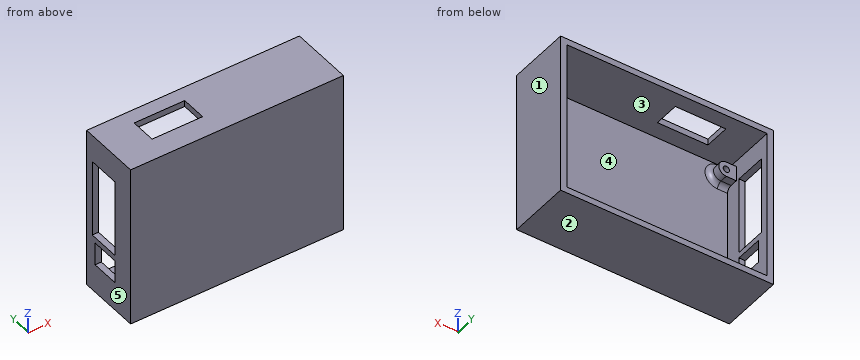
```python
from build123d import *

# Parameters (mm, degrees)
SKETCH_1_W          = 85
SKETCH_1_H          = 65
EXTRUDE_1_DEPTH     = 25
SHELL_1_T           = -2.5
SKETCH_2_R          = 3
SKETCH_2_R_2        = 1.25
EXTRUDE_2_DEPTH     = 5
SKETCH_3_W          = 20.2
SKETCH_3_H          = 10.2
CUT_EXTRUDE_1_DEPTH = 3.5
SKETCH_4_W          = 9.2
SKETCH_4_H          = 11.2
SKETCH_4_W_2        = 31
SKETCH_4_H_2        = 12.8
CUT_EXTRUDE_2_DEPTH = 3.5
FILLET_1_R          = 2


with BuildPart() as part:
    # 草图1 → 凸台-拉伸1 (new body)
    with BuildSketch(Plane(origin=(0, 0, 0), x_dir=(1, 0, 0), z_dir=(0, 1, 0))):
        Rectangle(SKETCH_1_W, SKETCH_1_H)
    extrude(amount=EXTRUDE_1_DEPTH)

    # 抽壳1
    shell_1_openings = [part.faces().sort_by_distance(p)[0] for p in [
        (0, 25, 0),
    ]]
    offset(amount=SHELL_1_T, openings=shell_1_openings, kind=Kind.INTERSECTION)

    # 草图2 → 凸台-拉伸2 (add)
    with BuildSketch(Plane(origin=(0, 2.5, 0), x_dir=(1, 0, 0), z_dir=(0, 1, 0))):
        with Locations((32.25, 24.75)):
            Circle(SKETCH_2_R)
        with Locations((32.25, 24.75)):
            Circle(SKETCH_2_R_2, mode=Mode.SUBTRACT)
        with Locations((32.25, -24.75)):
            Circle(SKETCH_2_R)
        with Locations((32.25, -24.75)):
            Circle(SKETCH_2_R_2, mode=Mode.SUBTRACT)
        with BuildLine():
            Line((-36, 27.75), (-40, 27.75))
            Line((-40, 27.75), (-40, 21.75))
            Line((-40, 21.75), (-36, 21.75))
            ThreePointArc((-36, 21.75), (-33, 24.75), (-36, 27.75))
        make_face()
        with Locations((-36, 24.75)):
            Circle(SKETCH_2_R_2, mode=Mode.SUBTRACT)
        with BuildLine():
            Line((-36, -21.75), (-40, -21.75))
            Line((-40, -21.75), (-40, -27.75))
            Line((-40, -27.75), (-36, -27.75))
            ThreePointArc((-36, -27.75), (-33, -24.75), (-36, -21.75))
        make_face()
        with Locations((-36, -24.75)):
            Circle(SKETCH_2_R_2, mode=Mode.SUBTRACT)
    extrude(amount=EXTRUDE_2_DEPTH)

    # 草图3 → 切除-拉伸1 (cut, through all)
    with BuildSketch(Plane(origin=(0, 0, 30), x_dir=(-1, 0, 0), z_dir=(0, 0, -1))):
        with Locations((17.5, 14.1)):
            Rectangle(SKETCH_3_W, SKETCH_3_H)
    extrude(amount=-CUT_EXTRUDE_1_DEPTH, mode=Mode.SUBTRACT)

    # 草图4 → 切除-拉伸2 (cut, through all)
    with BuildSketch(Plane(origin=(-40, 0, 0), x_dir=(0, 0, -1), z_dir=(1, 0, 0))):
        with Locations((16.4, 14.6)):
            Rectangle(SKETCH_4_W, SKETCH_4_H)
        with Locations((-6, 15.4)):
            Rectangle(SKETCH_4_W_2, SKETCH_4_H_2)
    extrude(amount=-CUT_EXTRUDE_2_DEPTH, mode=Mode.SUBTRACT)

    # 圆角1
    fillet_1_edges = [part.edges().sort_by_distance(p)[0] for p in [
        (29.25, 2.5, -24.75),
        (29.25, 2.5, 24.75),
        (-33, 2.5, -24.75),
        (-38, 2.5, -27.75),
        (-38, 2.5, -21.75),
        (-33, 2.5, 24.75),
        (-38, 2.5, 21.75),
        (-38, 2.5, 27.75),
    ]]
    fillet(fillet_1_edges, radius=FILLET_1_R)


solid = part.part
```
Check sheet for the modelled part. Datum: model origin and axes. Units: mm. Face numbers are marked on the shaded views. A direction names the side the tool comes from. Round coordinates to 2 decimals unless told otherwise and drop trailing zeros. Write each loop counter-clockwise with the first axis right and the second up, starting at its lowest first coordinate (ties: lowest second). Pieces come first, ordered by that corner, then holes. Notation, with made-up numbers: (86.25, 74.25) -> (123.25, 74.25) arc R23 ccw to (123.25, 99.25) -> close; hole circle Ø10 at (-31.75, -9.5). An arc over 180 degrees is marked (long way). Put each result on its own line as item: value.
(1) Sectioned sample at C-C (x = 8). Enter the section's corners in (y, z).
Values found:
outline: (0, -32.5) -> (25, -32.5) -> (25, -30) -> (2.5, -30) -> (2.5, 30) -> (25, 30) -> (25, 32.5) -> (0, 32.5) -> close
(2) Tool access check on the marked faces 4 and 5. Record the directions out of +Z, -Z, +X, -X, +Y, -Y that give a thin tool (end or side, any length) a straight path to the whole face; none if there is none.
Values found:
face 4: +Y
face 5: +Z, -Z, -X, +Y, -Y
(3) Sectioned sample at A-A (y = 15). Enter the section's corners in (x, z), plus the area to 3 significant figures.
Values found:
outline: (-42.5, -32.5) -> (42.5, -32.5) -> (42.5, 32.5) -> (-7.4, 32.5) -> (-7.4, 30) -> (40, 30) -> (40, -30) -> (-40, -30) -> (-40, -21) -> (-42.5, -21) -> close; (-42.5, -11.8) -> (-40, -11.8) -> (-40, -9.5) -> (-42.5, -9.5) -> close; (-42.5, 21.5) -> (-40, 21.5) -> (-40, 30) -> (-27.6, 30) -> (-27.6, 32.5) -> (-42.5, 32.5) -> close
area: 574 mm^2
(4) Go/stop test with flat-tipped pins: pin 1 Ø3 at (x, z) = (33.5, 24.5) entering from +Y; pin 2 Ø1.5 at (y, z) = (13, 13.5) entering from -X. Record where each tip stops, or that it passes through.
Values found:
pin 1: stops at y = 7.5
pin 2: stops at x = 40
(5) Mould release check, pull along X, two halves, no side actions. Record for the marked faces 1, 2 and 3: released by +X, released by -X, zero draft, split by the parting line, or undercut.
Values found:
face 1: released by +X
face 2: zero draft
face 3: undercut
(6) Material ranges on line 1 (Z direction, x = 32.25, y = 6.1); line 2 (X direction, y = 5.55, z = 24.75), recorded low to high.
Values found:
line 1: z = -32.5 to -30, -27.75 to -26, -23.5 to -21.75, 21.75 to 23.5, 26 to 27.75, 30 to 32.5
line 2: x = -42.5 to -37.25, -34.75 to -33, 29.25 to 31, 33.5 to 35.25, 40 to 42.5
(7) Sectioned sample at B-B (z = 9). Enter the section's corners in (x, y).
Values found:
outline: (-42.5, 0) -> (42.5, 0) -> (42.5, 25) -> (40, 25) -> (40, 2.5) -> (-40, 2.5) -> (-40, 9) -> (-42.5, 9) -> close; (-42.5, 21.8) -> (-40, 21.8) -> (-40, 25) -> (-42.5, 25) -> close
(8) Sectioned sample at D-D (z = -10.5). Enter the section's corners in (x, y), plus the area to 3 significant figures.
Values found:
outline: (-42.5, 0) -> (42.5, 0) -> (42.5, 25) -> (40, 25) -> (40, 2.5) -> (-40, 2.5) -> (-40, 25) -> (-42.5, 25) -> close
area: 325 mm^2
